from build123d import *

# Parameters (mm, degrees)
EXTRUDE_1_DEPTH     = 16
SKETCH_2_R          = 1.65
CUT_EXTRUDE_1_DEPTH = 22.412613105
FILLET_1_R          = 2


with BuildPart() as part:
    # 草图1 → 凸台-拉伸1 (new body)
    with BuildSketch(Plane.XY):
        with BuildLine():
            Line((-6.32455532, -1.5), (-13.5, -1.5))
            Line((-13.5, -1.5), (-13.5, -4))
            Line((-13.5, -4), (-7.5, -4))
            ThreePointArc((-7.5, -4), (0, -8.5), (7.5, -4))
            Line((7.5, -4), (13.5, -4))
            Line((13.5, -4), (13.5, -1.5))
            Line((13.5, -1.5), (6.32455532, -1.5))
            ThreePointArc((6.32455532, -1.5), (0, -6.5), (-6.32455532, -1.5))
        make_face()
    extrude(amount=EXTRUDE_1_DEPTH)

    # 草图2 → 切除-拉伸1 (cut, through all)
    with BuildSketch(Plane.XZ.offset(4)):
        with Locations(Location((-10.5, 8, 0), (0, 0, 270))):
            Circle(SKETCH_2_R)
        with Locations(Location((10.5, 8, 0), (0, 0, 270))):
            Circle(SKETCH_2_R)
    extrude(amount=-CUT_EXTRUDE_1_DEPTH, mode=Mode.SUBTRACT)

    # 圆角1
    fillet_1_edges = [part.edges().sort_by_distance(p)[0] for p in [
        (-13.5, -2.75, 16),
        (13.5, -2.75, 16),
        (13.5, -2.75, 0),
        (-13.5, -2.75, 0),
    ]]
    fillet(fillet_1_edges, radius=FILLET_1_R)


solid = part.part
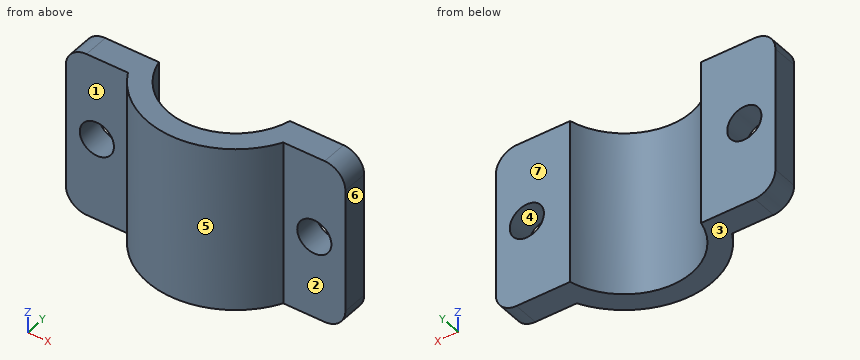
Read the model definition and answer for the solid it produces. Units are mm, in the model's axes. Face numbers are marked on the shaded views. A direction names the side the tool comes from. Give positions to 0.01 mm unless a question says otherwise; leave off trailing zeros. Loops run counter-clockwise (first coordinate to the right, second up) from the corner with the lowest first, then second, coordinate; pieces in that order, holes last. Notation, with made-up numbers: (12.5, 68.5) - (69.5, 68.5) arc R21 cw to (69.5, 92.5) - close; hole circle Ø11 at (84, 4). An arc over 180 degrees is marked (long way). Answer as CSV lines item,"result". Start each with the question number.
1) Find section A-A (x = -10.5). Write down the section's boundary in (y, z), then the cut area to 4 significant figures.
2) Each of these flat-tipped pins is pushed along its axis until it touches: pin 1 Ø2.5 at (x, z) = (-10.5, 8) entering from +Y; pin 2 Ø1.5 at (y, z) = (-7, 7) entering from -X; pin 3 Ø2 at (y, z) = (-6, 5.5) entering from -X; pin 4 Ø4 at (x, z) = (10.5, 8) entering from -Y. Where does it stop, or does it pass through?
3) Straight lines are drawn through the part: L1, parallel to X at y = -2.75, z = 8; L2, parallel to X at y = -2.6, z = 8; L3, parallel to Y at x = -12.5, z = 8.25. For each, find the intervals that lie inside material, in ascending order. Write a range as from..to.
4) Determine the mould class of the marked faces 4, 5, 6 and 7 for opening direction X: released by +X, released by -X, zero draft, split by the parting line, or undercut.
5) Find section D-D (y = -5.75). Write down the section's boundary in (x, z).
6) Find section C-C (z = 8). Write down the section's boundary in (x, y).
7) Find section B-B (y = -3). Write down the section's boundary in (x, z).
8) Which of the six approach directions +Z, -Z, +X, -X, +Y, -Y give full straight-line access (tool end or side, diameter ignored) to the marked faces 1, 2 and 3?
Findings below:
1,outline,"(-4, 0) - (-1.5, 0) - (-1.5, 6.35) - (-4, 6.35) - close; (-4, 9.65) - (-1.5, 9.65) - (-1.5, 16) - (-4, 16) - close"
1,area,"31.75 mm^2"
2,pin 1,"through"
2,pin 2,"x = -5.76"
2,pin 3,"x = -6.87"
2,pin 4,"y = -4"
3,L1,"-13.5..-12.15, -8.85..-5.89, 5.89..8.85, 12.15..13.5"
3,L2,"-13.5..-12.15, -8.85..-5.96, 5.96..8.85, 12.15..13.5"
3,L3,"-4..-1.5"
4,face 4,"undercut"
4,face 5,"split by the parting line"
4,face 6,"released by +X"
4,face 7,"zero draft"
5,outline,"(-6.26, 0) - (-3.03, 0) - (-3.03, 16) - (-6.26, 16) - close; (3.03, 0) - (6.26, 0) - (6.26, 16) - (3.03, 16) - close"
6,outline,"(-13.5, -4) - (-12.15, -4) - (-12.15, -1.5) - (-13.5, -1.5) - close; (-8.85, -4) - (-7.5, -4) arc R8.5 ccw to (7.5, -4) - (8.85, -4) - (8.85, -1.5) - (6.32, -1.5) arc R6.5 cw to (-6.32, -1.5) - (-8.85, -1.5) - close; (12.15, -4) - (13.5, -4) - (13.5, -1.5) - (12.15, -1.5) - close"
7,outline,"(-13.5, 2) arc R2 ccw to (-11.5, 0) - (-5.77, 0) - (-5.77, 16) - (-11.5, 16) arc R2 ccw to (-13.5, 14) - close; (5.77, 0) - (11.5, 0) arc R2 ccw to (13.5, 2) - (13.5, 14) arc R2 ccw to (11.5, 16) - (5.77, 16) - close; hole circle Ø3.3 at (-10.5, 8); hole circle Ø3.3 at (10.5, 8)"
8,face 1,"+Z, -Z, -X, -Y"
8,face 2,"+Z, -Z, +X, -Y"
8,face 3,"-Z, +X, -X, +Y, -Y"
